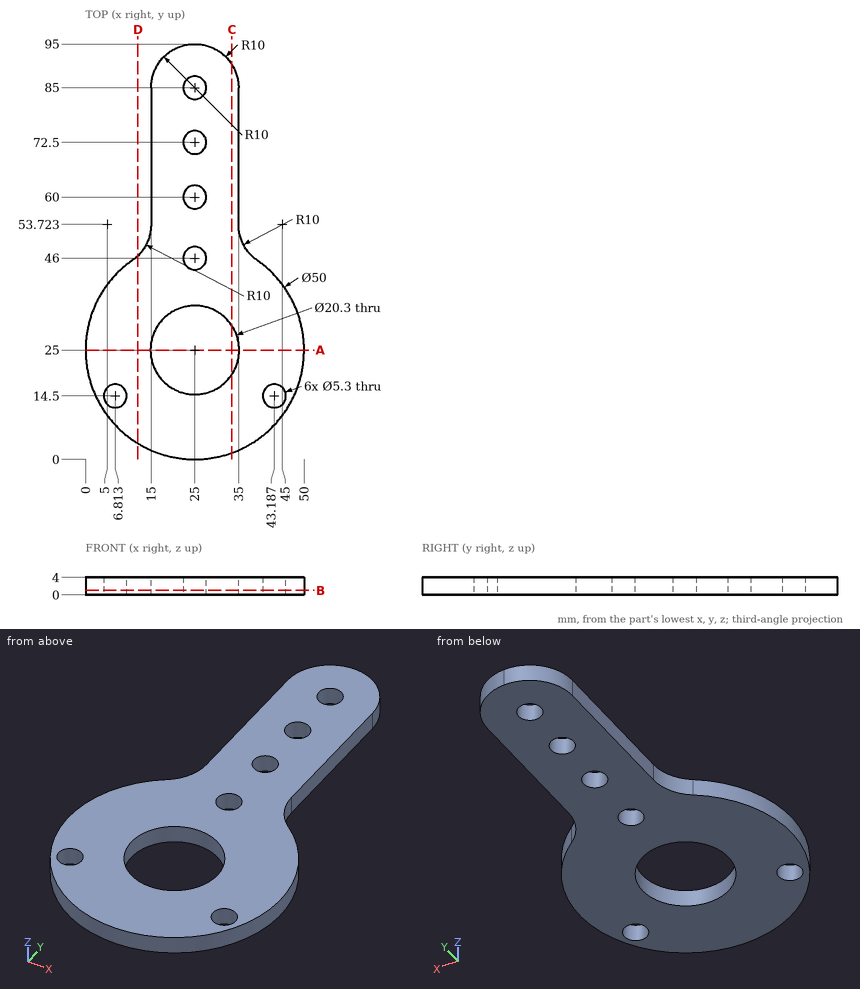
Source: three-view drawing plus pictorial views. Frame: mm from the lowest corner of the part. Round coordinates to 2 decimals unless told otherwise and drop trailing zeros. Loops run counter-clockwise (first coordinate to the right, second up) from the corner with the lowest first, then second, coordinate; pieces in that order, holes last. Notation, with made-up numbers: M 56.25,38.5 L 106.25,38.5 A33 cw 106.25,69.5 Z; hole C -3.75,-7 d11. An arc over 180 degrees is marked long. Answer as CSV lines item,"result".
Q1. Cut plane D-D (x = 12). Return the cut outline in (y, z) (1 decimal), plus the area to 3 significant figures.
Verdict:
outline,"M 3.6,0 L 46.6,0 L 46.6,4 L 3.6,4 Z"
area,"172 mm^2"
Q2. Cut plane B-B (z = 1). Count the separate pieces of the cut face and the enclosed holes in it, plus the area to 3 significant figures.
Verdict:
separate pieces,"1"
enclosed holes,"7"
area,"2,390 mm^2"
Q3. Cut plane C-C (x = 33.5). Return the cut outline in (y, z), plus the area to 3 significant figures.
Verdict:
outline,"M 1.49,0 L 19.45,0 L 19.45,4 L 1.49,4 Z; M 30.55,0 L 90.27,0 L 90.27,4 L 30.55,4 Z"
area,"311 mm^2"
Q4. Cut plane A-A (y = 25). Return the cut outline in (x, z).
Verdict:
outline,"M 0,0 L 14.85,0 L 14.85,4 L 0,4 Z; M 35.15,0 L 50,0 L 50,4 L 35.15,4 Z"
Q5. Line query: line 1 along Y through (x, z) = (25, 0.3); line 2 along Y through (x, z) = (30, 3.35) (1 decimal); line 3 along Y through (x, z) = (22, 1.3) (1 decimal). Output: solid intervals per line, ascending.
Verdict:
line 1,"y = 0 to 14.85, 35.15 to 43.35, 48.65 to 57.35, 62.65 to 69.85, 75.15 to 82.35, 87.65 to 95"
line 2,"y = 0.5 to 16.2, 33.8 to 93.7"
line 3,"y = 0.2 to 15.3, 34.7 to 94.5"
Q6. Contact query for flat-ended pins moving along their axis: pin 1 (1 mm diameter, centred on y = 56.5, z = 0.5, fed in from +X); pin 2 (4 mm diameter, centred on x = 25, y = 85, fed in from +Z); pin 3 (7 mm diameter, centred on x = 25, y = 46, fed in from -Z); pin 4 (1.2 mm diameter, centred on y = 74, z = 1, fed in from -X). Output: stop coordinate, or through.
Verdict:
pin 1,"stops at x = 35"
pin 2,"passes through"
pin 3,"stops at z = 0"
pin 4,"stops at x = 15"
